The model under review builds one solid part; all positions refer to its coordinate system, in mm. A direction names the side the tool comes from. Coordinates: 2 decimals unless noted, no trailing zeros. Write each loop counter-clockwise with the first axis right and the second up, starting at its lowest first coordinate (ties: lowest second). Pieces come first, ordered by that corner, then holes.
```python
from build123d import *
from build123d.topology import SkipClean

# Parameters (mm, degrees)
SKETCH2_R           = 6.575
BOSS_EXTRUDE1_DEPTH = 5
SKETCH4_R           = 2.125
BOSS_EXTRUDE3_DEPTH = 2
SKETCH5_R           = 1.8
BOSS_EXTRUDE4_DEPTH = 2
BOSS_EXTRUDE5_DEPTH = 10
CUT_EXTRUDE1_START  = -10
CUT_EXTRUDE1_DEPTH  = 10
CUT_EXTRUDE2_DEPTH  = 10


with BuildPart() as part:
    # Sketch2 → Boss-Extrude1 (new body)
    with BuildSketch(Plane.XY):
        with BuildLine():
            Line((-20, 0), (-20, -97))
            ThreePointArc((-20, -97), (0, -117), (20, -97))
            Line((20, -97), (20, 0))
            ThreePointArc((20, 0), (0, 20), (-20, 0))
        make_face()
        Circle(SKETCH2_R, mode=Mode.SUBTRACT)
    extrude(amount=BOSS_EXTRUDE1_DEPTH)

    # Sketch4 → Boss-Extrude3 (add)
    with BuildSketch(Plane.XY.offset(5)):
        with Locations((-8, 8)):
            Circle(SKETCH4_R)
        with Locations((8, 8)):
            Circle(SKETCH4_R)
        with Locations((8, -8)):
            Circle(SKETCH4_R)
        with Locations((-8, -8)):
            Circle(SKETCH4_R)
    extrude(amount=BOSS_EXTRUDE3_DEPTH)

    # Sketch5 → Boss-Extrude4 (add)
    with BuildSketch(Plane.XY.offset(7)):
        with Locations((-8, 8)):
            Circle(SKETCH5_R)
        with Locations((8, 8)):
            Circle(SKETCH5_R)
        with Locations((8, -8)):
            Circle(SKETCH5_R)
        with Locations((-8, -8)):
            Circle(SKETCH5_R)
    extrude(amount=BOSS_EXTRUDE4_DEPTH)

    # Sketch6 → Boss-Extrude5 (add)
    with BuildSketch(Plane.XY.offset(5)):
        with BuildLine():
            Line((20, -97), (20, 0))
            ThreePointArc((20, 0), (0, 20), (-20, 0))
            Line((-20, 0), (-20, -97))
            ThreePointArc((-20, -97), (0, -117), (20, -97))
        make_face()
        with BuildLine():
            Line((-19, 0), (-19, -97))
            ThreePointArc((-19, -97), (0, -116), (19, -97))
            Line((19, -97), (19, 0))
            ThreePointArc((19, 0), (0, 19), (-19, 0))
        make_face(mode=Mode.SUBTRACT)
    extrude(amount=BOSS_EXTRUDE5_DEPTH)

    # Sketch7 → Cut-Extrude1 (cut)
    with BuildSketch(Plane.XY.offset(5).offset(CUT_EXTRUDE1_START)):
        with BuildLine():
            Line((-10.125, 8), (-10.125, -8))
            ThreePointArc((-10.125, -8), (-9.50260191, -6.49739809), (-8, -5.875))
            Line((-8, -5.875), (-8, 5.875))
            ThreePointArc((-8, 5.875), (-9.50260191, 6.49739809), (-10.125, 8))
        make_face()
        with BuildLine():
            Line((-8, -10.125), (8, -10.125))
            ThreePointArc((8, -10.125), (6.49739809, -9.50260191), (5.875, -8))
            Line((5.875, -8), (-5.875, -8))
            ThreePointArc((-5.875, -8), (-6.49739809, -9.50260191), (-8, -10.125))
        make_face()
        with BuildLine():
            Line((10.125, -8), (10.125, 8))
            ThreePointArc((10.125, 8), (9.50260191, 6.49739809), (8, 5.875))
            Line((8, 5.875), (8, -5.875))
            ThreePointArc((8, -5.875), (9.50260191, -6.49739809), (10.125, -8))
        make_face()
        with BuildLine():
            Line((8, 10.125), (-8, 10.125))
            ThreePointArc((-8, 10.125), (-6.49739809, 9.50260191), (-5.875, 8))
            Line((-5.875, 8), (5.875, 8))
            ThreePointArc((5.875, 8), (6.49739809, 9.50260191), (8, 10.125))
        make_face()
    extrude(amount=CUT_EXTRUDE1_DEPTH, mode=Mode.SUBTRACT)

    # Sketch10 → Cut-Extrude2 (cut)
    with SkipClean():  # the faces are left unmerged after this step: merging them gives an invalid solid
        with BuildSketch(Plane(origin=(0, 0, 0), x_dir=(-1, 0, 0), z_dir=(0, 0, -1))):
            with BuildLine():
                Line((-8, 10.125), (-11.181980515, 13.306980515))
                ThreePointArc((-11.181980515, 13.306980515), (0, 17.938708499), (11.181980515, 13.306980515))
                Line((11.181980515, 13.306980515), (8, 10.125))
                Line((8, 10.125), (-8, 10.125))
            make_face()
            with BuildLine():
                Line((-10.125, 8), (-13.306980515, 11.181980515))
                ThreePointArc((-13.306980515, 11.181980515), (-17.938708499, 0), (-13.306980515, -11.181980515))
                Line((-13.306980515, -11.181980515), (-10.125, -8))
                Line((-10.125, -8), (-10.125, 8))
            make_face()
            with BuildLine():
                Line((10.125, 8), (13.306980515, 11.181980515))
                ThreePointArc((13.306980515, 11.181980515), (17.938708499, 0), (13.306980515, -11.181980515))
                Line((13.306980515, -11.181980515), (10.125, -8))
                Line((10.125, -8), (10.125, 8))
            make_face()
            with BuildLine():
                Line((8, -10.125), (11.181980515, -13.306980515))
                ThreePointArc((11.181980515, -13.306980515), (0, -17.938708499), (-11.181980515, -13.306980515))
                Line((-11.181980515, -13.306980515), (-8, -10.125))
                Line((-8, -10.125), (8, -10.125))
            make_face()
        extrude(amount=-CUT_EXTRUDE2_DEPTH, mode=Mode.SUBTRACT)


solid = part.part
```
Item 1: Take a section at A-A, the plane x = 0. Write out the cut boundary in (y, z) (3 decimals), plus the area to 3 significant figures.
Solved:
outline: (-117, 0) - (-17.939, 0) - (-17.939, 5) - (-116, 5) - (-116, 15) - (-117, 15) - close; (-8, 0) - (-6.575, 0) - (-6.575, 5) - (-8, 5) - close; (6.575, 0) - (8, 0) - (8, 5) - (6.575, 5) - close; (17.939, 0) - (20, 0) - (20, 15) - (19, 15) - (19, 5) - (17.939, 5) - close
area: 540 mm2
Item 2: To check wall thickness, follow line 1 along Y through (x, z) = (0, 3.8) (3 decimals); line 2 along X through (y, z) = (-91, 12.5); line 3 along Y through (x, z) = (9, 3.25) (3 decimals). State the ranges of each line that lie inside material, in increasing order.
Solved:
line 1: y = -117 to -17.939, -8 to -6.575, 6.575 to 8, 17.939 to 20
line 2: x = -20 to -19, 19 to 20
line 3: y = -114.861 to -15.128, -11.125 to -6.125, 6.125 to 11.125, 15.128 to 17.861
Item 3: Take a section at B-B, the plane z = 11. Write out the cut boundary in (x, y).
Solved:
outline: (-20, -97) arc R20 ccw to (20, -97) - (20, 0) arc R20 ccw to (-20, 0) - close; hole (-19, -97) arc R19 ccw to (19, -97) - (19, 0) arc R19 ccw to (-19, 0) - close
Item 4: Mouldability with a two-part tool opening along X and no side actions: class faces 1 (the face through (-8, 0, 2)), 2 (the face through (20, -49, 7)), 3 (the face through (0, 20, 7)) as pulls with the +X half, pulls with the -X half, needs draft (parallel to the pull), parting line crosses it, or undercut.
Solved:
face 1: undercut
face 2: pulls with the +X half
face 3: parting line crosses it
Item 5: For pin 1 (1.5 mm diameter, centred on y = 5, z = 5, fed in from +X); pin 2 (2 mm diameter, centred on x = 8, y = 9, fed in from +Z); pin 3 (5 mm diameter, centred on x = 3.5, y = -3, fed in from +Z), all flat-tipped, find the tip position at first contact; note any pin that passes through.
Solved:
pin 1: stops at x = 19.54
pin 2: stops at z = 9
pin 3: stops at z = 5
Item 6: Machinability: for faces 4 (the face through (8, -8, 9)), 5 (the face through (17.938, 0.174, 2.465)), which of the approach directions +Z, -Z, +X, -X, +Y, -Y give a long, thin tool a straight path to every point of the face, cutting with its end or side? Answer none if there is none.
Solved:
face 4: +Z
face 5: +Z, -Z
Item 7: Take a section at C-C, the plane y = -51. Write out the cut boundary in (x, z).
Solved:
outline: (-20, 0) - (20, 0) - (20, 15) - (19, 15) - (19, 5) - (-19, 5) - (-19, 15) - (-20, 15) - close
